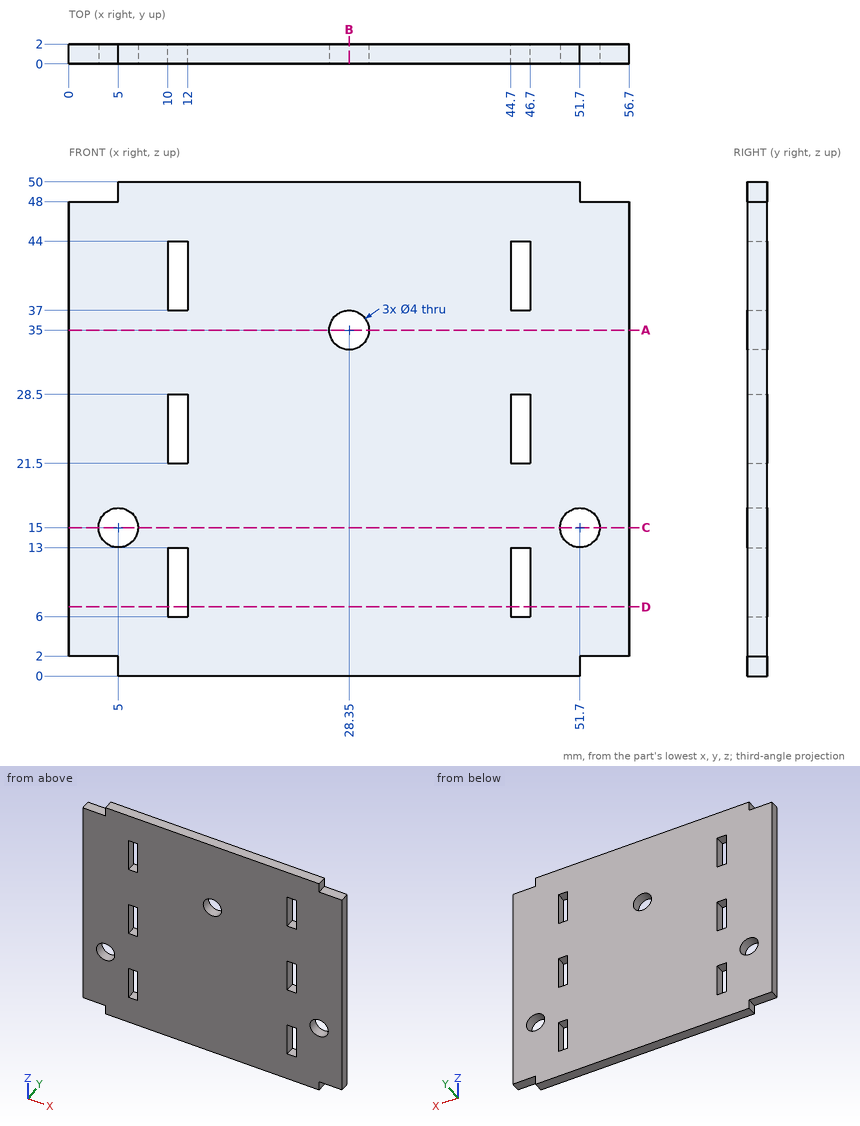
Source: three-view drawing plus pictorial views. Frame: mm from the lowest corner of the part. Round coordinates to 2 decimals unless told otherwise and drop trailing zeros. Loops run counter-clockwise (first coordinate to the right, second up) from the corner with the lowest first, then second, coordinate; pieces in that order, holes last. Notation, with made-up numbers: (27.5, 88) -> (72.5, 88) arc R31 cw to (72.5, 113) -> close; hole circle Ø5 at (12.5, 68.5). An arc over 180 degrees is marked (long way). Use one line per item in the form item = value.
Item 1: Contact query for flat-ended pins moving along their axis: pin 1 Ø1 at (x, y) = (55, 1) entering from +Z; pin 2 Ø1 at (y, z) = (1, 1) entering from -X; pin 3 Ø3.5 at (x, z) = (28.35, 35) entering from +Y. Output: stop coordinate, or through.
Evaluation:
pin_1 = 48
pin_2 = 5
pin_3 = through
Item 2: Cut plane A-A on z = 35. Output: boundary loops of the cut face in (x, y), then the cut area to 3 significant figures.
Evaluation:
outline = (0, 0) -> (26.35, 0) -> (26.35, 2) -> (0, 2) -> close; (30.35, 0) -> (56.7, 0) -> (56.7, 2) -> (30.35, 2) -> close
area = 105 mm2
Item 3: Cut plane C-C on z = 15. Output: boundary loops of the cut face in (x, y).
Evaluation:
outline = (0, 0) -> (3, 0) -> (3, 2) -> (0, 2) -> close; (7, 0) -> (49.7, 0) -> (49.7, 2) -> (7, 2) -> close; (53.7, 0) -> (56.7, 0) -> (56.7, 2) -> (53.7, 2) -> close
Item 4: Cut plane D-D on z = 7. Output: boundary loops of the cut face in (x, y), then the cut area to 3 significant figures.
Evaluation:
outline = (0, 0) -> (10, 0) -> (10, 2) -> (0, 2) -> close; (12, 0) -> (44.7, 0) -> (44.7, 2) -> (12, 2) -> close; (46.7, 0) -> (56.7, 0) -> (56.7, 2) -> (46.7, 2) -> close
area = 105 mm2
Item 5: Cut plane B-B on x = 28.35. Output: boundary loops of the cut face in (y, z), then the cut area to 3 significant figures.
Evaluation:
outline = (0, 0) -> (2, 0) -> (2, 33) -> (0, 33) -> close; (0, 37) -> (2, 37) -> (2, 50) -> (0, 50) -> close
area = 92.0 mm2
Item 6: Material intervals for probe 1 along X at (y, z) = (0.3, 28); probe 2 along X at (y, z) = (0.75, 15); probe 3 along Z at (x, y) = (46, 0.9), sorted ascending.
Evaluation:
probe_1 = 0 to 10, 12 to 44.7, 46.7 to 56.7
probe_2 = 0 to 3, 7 to 49.7, 53.7 to 56.7
probe_3 = 0 to 6, 13 to 21.5, 28.5 to 37, 44 to 50
